Geometry: final body of the model. Coordinates: model frame, mm. Give positions to 0.01 mm unless a question says otherwise; leave off trailing zeros. Loops run counter-clockwise (first coordinate to the right, second up) from the corner with the lowest first, then second, coordinate; pieces in that order, holes last. Notation, with made-up numbers: (40, -22) - (51, -22) arc R21 cw to (51, 5) - close; hole circle Ø1 at (-35, 36.5). An arc over 180 degrees is marked (long way). Use CSV: the item, a comma, the result in double quotes. Start each with the question number.
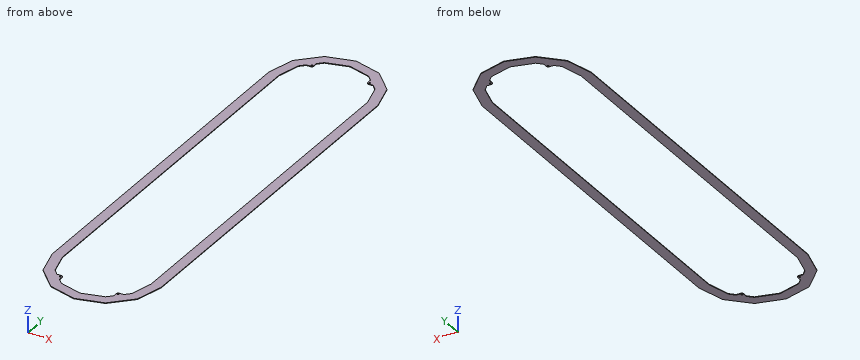
```python
from build123d import *

# Parameters (mm, degrees)
F1_DEPTH = 1.5875
F3_DEPTH = 1.5875
F4_R     = 2.15265
F5_DEPTH = 1.5875


with BuildPart() as f1:
    # F0 (on Top) → F1 (new body)
    with BuildSketch(Plane.XY):
        Polygon((279.4, -920.6744858), (279.4, 0), (260.6837489087, 69.85), (209.55, 120.9837489087), (139.7, 139.7), (69.85, 120.9837489087), (18.7162510913, 69.85), (0, 0), (0, -920.6744858), (18.7162510913, -990.5244858), (69.85, -1041.6582347087), (139.7, -1060.3744858), (209.55, -1041.6582347087), (260.6837489087, -990.5244858), align=None)
    extrude(amount=F1_DEPTH)

    # F2 (on face) → F3 (cut, through all)
    with BuildSketch(Plane.XY.offset(1.5875)):
        Polygon((253.1039850176, -920.6744858), (253.1039850176, 0), (237.9107319156, 56.7019925088), (196.4019925088, 98.2107319156), (139.7, 113.4039850176), (82.9980074912, 98.2107319156), (41.4892680844, 56.7019925088), (26.2960149824, 0), (26.2960149824, -920.6744858), (41.4892680844, -977.3764783088), (82.9980074912, -1018.8852177156), (139.7, -1034.0784708176), (196.4019925088, -1018.8852177156), (237.9107319156, -977.3764783088), align=None)
    extrude(amount=-F3_DEPTH, mode=Mode.SUBTRACT)

    # F4 (on face) → F5 (join, through all)
    with BuildSketch(Plane.XY.offset(1.5875)):
        with BuildLine():
            Line((225.2864582576, 69.3262661668), (209.0262661668, 85.5864582576))
            Line((209.0262661668, 85.5864582576), (209.0262661668, 74.0887661668))
            ThreePointArc((209.0262661668, 74.0887661668), (210.4211701214, 70.7211701214), (213.7887661668, 69.3262661668))
            Line((213.7887661668, 69.3262661668), (225.2864582576, 69.3262661668))
        make_face()
        with Locations((213.7887661668, 74.0887661668)):
            Circle(F4_R, mode=Mode.SUBTRACT)
        with BuildLine():
            ThreePointArc((65.6112338332, 69.3262661668), (68.9788298786, 70.7211701214), (70.3737338332, 74.0887661668))
            Line((70.3737338332, 74.0887661668), (70.3737338332, 85.5864582576))
            Line((70.3737338332, 85.5864582576), (54.1135417424, 69.3262661668))
            Line((54.1135417424, 69.3262661668), (65.6112338332, 69.3262661668))
        make_face()
        with Locations((65.6112338332, 74.0887661668)):
            Circle(F4_R, mode=Mode.SUBTRACT)
        with BuildLine():
            Line((65.6112338332, -990.0007519668), (54.1135417424, -990.0007519668))
            Line((54.1135417424, -990.0007519668), (70.3737338332, -1006.2609440576))
            Line((70.3737338332, -1006.2609440576), (70.3737338332, -994.7632519668))
            ThreePointArc((70.3737338332, -994.7632519668), (68.9788298786, -991.3956559214), (65.6112338332, -990.0007519668))
        make_face()
        with Locations((65.6112338332, -994.7632519668)):
            Circle(F4_R, mode=Mode.SUBTRACT)
        with BuildLine():
            Line((209.0262661668, -1006.2609440576), (225.2864582576, -990.0007519668))
            Line((225.2864582576, -990.0007519668), (213.7887661668, -990.0007519668))
            ThreePointArc((213.7887661668, -990.0007519668), (210.4211701214, -991.3956559214), (209.0262661668, -994.7632519668))
            Line((209.0262661668, -994.7632519668), (209.0262661668, -1006.2609440576))
        make_face()
        with Locations((213.7887661668, -994.7632519668)):
            Circle(F4_R, mode=Mode.SUBTRACT)
    extrude(amount=-F5_DEPTH)


solid = f1.part
```
Item 1: Section C-C (z = 1.2). Give the number of separate pieces and of enclosed holes in the cut face, plus the area to 3 significant figures.
Item 2: Pin query (flat end, axial travel): pin 1 Ø5 at (x, y) = (65.61, -994.76) entering from +Z; pin 2 Ø3.5 at (x, y) = (213.79, 74.09) entering from +Z; pin 3 Ø0.8 at (x, z) = (60, 0.5) entering from +Y; pin 4 Ø0.8 at (y, z) = (-1001.5, 1) entering from -X. Return the tip coordinate at first contact, or that it passes through.
Item 3: Ray query, probe 1 along X at (y, z) = (-648.5, 0.5); probe 2 along Y at (x, z) = (215.5, 1.1); probe 3 along Y at (x, z) = (212, 1.4). Return the intervals inside material, ascending.
Item 4: Section B-B (x = 123). Output: boundary loops of the cut face in (y, z).
Item 5: Section A-A (y = -104). Output: boundary loops of the cut face in (x, z).
Outcome:
1,separate pieces,"1"
1,enclosed holes,"5"
1,area,"68,800 mm2"
2,pin 1,"stops at z = 1.59"
2,pin 2,"passes through"
2,pin 3,"stops at y = 111.53"
2,pin 4,"stops at x = 29.29"
3,probe 1,"x = 0 to 26.3, 253.1 to 279.4"
3,probe 2,"y = -1035.71 to -996.07, -993.46 to -990, 69.33 to 72.78, 75.39 to 115.03"
3,probe 3,"y = -1039.21 to -995.96, -993.57 to -990.35, 69.67 to 72.89, 75.29 to 118.53"
4,outline,"(-1055.9, 0) - (-1029.6, 0) - (-1029.6, 1.59) - (-1055.9, 1.59) - close; (108.93, 0) - (135.23, 0) - (135.23, 1.59) - (108.93, 1.59) - close"
5,outline,"(0, 0) - (26.3, 0) - (26.3, 1.59) - (0, 1.59) - close; (253.1, 0) - (279.4, 0) - (279.4, 1.59) - (253.1, 1.59) - close"
